Read the model definition and answer for the solid it produces. Units are mm, in the model's axes. A direction names the side the tool comes from. Coordinates: 2 decimals unless noted, no trailing zeros. Write each loop counter-clockwise with the first axis right and the second up, starting at its lowest first coordinate (ties: lowest second). Pieces come first, ordered by that corner, then holes.
Item 1: Determine the mould class of faces 4 (the face through (-13, 120, 2)), 5 (the face through (30, 147.049, 2)), 6 (the face through (22, -1, 2)) for opening direction X: released by +X, released by -X, zero draft, split by the parting line, or undercut.
Item 2: Each of these flat-tipped pins is pushed along its axis until it touches: P1, Ø1, axis at x = 18.5, z = 1, coming from the +Y side; P2, Ø0.9, axis at y = 145.5, z = 1.5, coming from the +X side; P3, Ø1.5, axis at y = 138.5, z = 1, coming from the -X side. Where does it stop, or does it pass through?
Item 3: A tool of negligible diameter and unlimited length cuts with its end or side. For faces 1 (the face through (-10, 137, 1)), 2 (the face through (39, 29.049, 2)), 3 (the face through (6, 146, 2)), from which of +Z, -Z, +X, -X, +Y, -Y can it reach the whole face along a straight path? Write none if from no direction.
Item 4: Straight lines are drawn through the part: probe 1 along Y at (x, z) = (23, 1.9); probe 2 along X at (y, z) = (90, 1.35); probe 3 along Y at (x, z) = (14, 1.3). For each, find the intervals that lie inside material, in ascending order.
Item 5: Section A-A (x = 14) is taken. Give the vertices of the cut face in (y, z).
Item 6: Section B-B (z = 2.15) is taken. State how many separate pieces and enclosed holes the cut face has, then the cut area to 3 significant figures.
Item 7: Section C-C (y = 69.5) is taken. Give the vertices of the cut face in (x, z).
Autodesk Inventor part; units mm, degrees
ref_plane "YZ Plane" through (0, 0, 0) normal (1, 0, 0) x (0, 1, 0)
ref_plane "XZ Plane" through (0, 0, 0) normal (0, 1, 0) x (-1, 0, 0)
ref_plane "XY Plane" through (0, 0, 0) normal (0, 0, 1) x (1, 0, 0)
sketch "Sketch1" plane through (0, 0, 0) normal (0, 0, 1) x (1, 0, 0)
  circle A0 centre (23, 103.0491) radius 1.5
  circle A1 centre (5, 103.0491) radius 1.5
  circle A2 centre (23, 136.0491) radius 1.5
  line L0 (-10, 144.0491) -> (38, 144.0491)
  line L1 (38, 144.0491) -> (38, -2.9509)
  line L2 (38, -2.9509) -> (-10, -2.9509)
  line L3 (-10, -2.9509) -> (-10, 144.0491)
  circle A3 centre (5, 136.0491) radius 1.5
  circle A4 centre (14, 126.5491) radius 3.5
  point P0 (0, 0)
  point P1 (14, 22.75)
  dimension "d10" = 3
  dimension "d12" = 3
  dimension "d13" = 3
  dimension "d14" = 3
  dimension "d15" = 33
  dimension "d16" = 18
  dimension "d17" = 18
  dimension "d18" = 33
  dimension "d19" = 15
  dimension "d20" = 8
  dimension "d21" = 15
  dimension "d22" = 147
  dimension "d25" = 7
  dimension "d26" = 9.5
  dimension "d27" = 9
  dimension "d28" = 9
  dimension "d29" = 2.9509
  dimension "d30" = 10
  dimension "d31" = 0
extrude "Extrusion1" add sketch "Sketch1" along normal blind 3
sketch "Sketch2" plane through (0, 0, 3) normal (0, 0, 1) x (1, 0, 0)
  line L0 (-10, 144.0491) -> (-10, -2.9509)
  line L1 (38, -2.9509) -> (38, 144.0491)
  line L2 (-10, 128.0491) -> (-13, 128.0491)
  line L3 (-13, 128.0491) -> (-13, 112.0491)
  line L4 (-13, 112.0491) -> (-10, 112.0491)
  line L5 (-10, 112.0491) -> (-10, 128.0491)
  line L6 (38, 128.0491) -> (41, 128.0491)
  line L7 (41, 128.0491) -> (41, 112.0491)
  line L8 (41, 112.0491) -> (38, 112.0491)
  line L9 (38, 112.0491) -> (38, 128.0491)
  line L10 (-10, 29.0491) -> (-13, 29.0491)
  line L11 (-13, 29.0491) -> (-13, 13.0491)
  line L12 (-13, 13.0491) -> (-10, 13.0491)
  line L13 (-10, 13.0491) -> (-10, 29.0491)
  line L14 (38, 29.0491) -> (41, 29.0491)
  line L15 (41, 29.0491) -> (41, 13.0491)
  line L16 (41, 13.0491) -> (38, 13.0491)
  line L17 (38, 13.0491) -> (38, 29.0491)
  line L18 (-10, -2.9509) -> (38, -2.9509)
  line L19 (38, 144.0491) -> (-10, 144.0491)
  line L20 (6, 144.0491) -> (22, 144.0491)
  line L21 (22, 144.0491) -> (22, 147.0491)
  line L22 (22, 147.0491) -> (6, 147.0491)
  line L23 (6, 147.0491) -> (6, 144.0491)
  line L24 (6, 144.0491) -> (-10, 144.0491)
  line L25 (-10, 144.0491) -> (-10, 147.0491)
  line L26 (-10, 147.0491) -> (6, 147.0491)
  line L27 (6, 147.0491) -> (6, 144.0491)
  line L28 (22, 144.0491) -> (38, 144.0491)
  line L29 (38, 144.0491) -> (38, 147.0491)
  line L30 (38, 147.0491) -> (22, 147.0491)
  line L31 (22, 147.0491) -> (22, 144.0491)
  point P0 (0, 0)
  point P1 (-11.5, 13.0491)
  point P2 (-10, 112.0491)
  point P3 (38, 112.0491)
  point P4 (22, 147.0491)
  point P5 (22, 144.0491)
  point P6 (-10, 144.0491)
  point P7 (6, 147.0491)
  dimension "d36" = 3
  dimension "d37" = 3
  dimension "d39" = 16
  dimension "d40" = 16
  dimension "d41" = 16
  dimension "d42" = 0
  dimension "d50" = 16
  dimension "d51" = 16
  dimension "d52" = 3
  dimension "d53" = 3
  dimension "d56" = 16
extrude "Extrusion2" add sketch "Sketch2" against normal blind 3 contours L25 L26 L23 L19 | L0 L4 L3 L2 | L21 L30 L29 L19 | L0 L12 L11 L10 | L6 L7 L8 L1 | L14 L15 L16 L1
sketch "Sketch4" plane through (0, 0, 3) normal (0, 0, 1) x (1, 0, 0)
  line L0 (-10, -2.9509) -> (38, -2.9509)
  line L1 (6, -2.9509) -> (22, -2.9509)
  line L2 (22, -2.9509) -> (22, 0.0491)
  line L3 (22, 0.0491) -> (6, 0.0491)
  line L4 (6, 0.0491) -> (6, -2.9509)
  line L5 (22, 144.0491) -> (6, 144.0491)
  line L6 (6, 144.0491) -> (6, 147.0491)
  point P0 (0, 0)
extrude "Extrusion4" cut sketch "Sketch4" against normal blind 3
equation "\"BendRadius\" = Thickness"
equation "\"BendReliefWidth\" = Thickness"
equation "\"BendReliefDepth\" = 0.5 * Thickness"
equation "\"CornerReliefSize\" = 4 * Thickness"
equation "\"MinimumRemnant\" = 2 * Thickness"
equation "\"TransitionRadius\" = BendRadius"
equation "\"JacobiRadiusSize\" = BendRadius"
equation "\"GapSize\" = Thickness"
properties part number "side plate" material "Hardboard"
Established:
1. face 4: released by -X
1. face 5: zero draft
1. face 6: undercut
2. P1: stops at y = 144.05
2. P2: stops at x = 38
2. P3: stops at x = -10
3. face 1: +Z, -Z, -X, +Y
3. face 2: +Z, -Z, +X
3. face 3: +Z, -Z, +Y
4. probe 1: y = -2.95 to 101.55, 104.55 to 134.55, 137.55 to 147.05
4. probe 2: x = -10 to 38
4. probe 3: y = 0.05 to 123.05, 130.05 to 144.05
5. outline: (0.05, 0) - (123.05, 0) - (123.05, 3) - (0.05, 3) - close; (130.05, 0) - (144.05, 0) - (144.05, 3) - (130.05, 3) - close
6. separate pieces: 1
6. enclosed holes: 5
6. area: 7,230 mm2
7. outline: (-10, 0) - (38, 0) - (38, 3) - (-10, 3) - close
